Source: CAD feature listing. Evaluate the final solid. Frame: model axes, mm. A direction names the side the tool comes from. Coordinates: 2 decimals unless noted, no trailing zeros. Loops run counter-clockwise (first coordinate to the right, second up) from the corner with the lowest first, then second, coordinate; pieces in that order, holes last. Notation, with made-up numbers: (-12, 21) -> (30, 21) arc R23 cw to (30, 54) -> close; hole circle Ø4 at (21.5, 47). An arc over 180 degrees is marked (long way). Answer as a JSON object with one key per item and string values. Group by question number.
from build123d import *

# Parameters (mm, degrees)
F1_DEPTH = 87.558992
F2_W     = 23.463726
F2_H     = 36.116287
F3_DEPTH = 159.944564


with BuildPart() as f1:
    # F0 (on Top) → F1 (new body)
    with BuildSketch(Plane.XY):
        Polygon((52.528806, 32.23221), (0, 21.399237), (-38.256936, -12.692079), (9.787939, -27.863212), align=None)
    extrude(amount=F1_DEPTH)

    # F2 (on face) → F3 (join)
    with BuildSketch(Plane(origin=(-10.628911, 11.927659, 0), x_dir=(-0.746584, -0.665292, 0), z_dir=(-0.665292, 0.746584, 0))):
        with Locations((9.666294, 53.462007)):
            Rectangle(F2_W, F2_H)
    extrude(amount=F3_DEPTH)


solid = f1.part
1. Mould query, pull axis X, two halves, no side actions, for faces 3 (the face through (26.63, 26.89, 43.17)), 4 (the face through (-70, 64, 35.404)), 5 (the face through (-14.57, -20.17, 43.17)). Classes: pulls with the +X half, pulls with the -X half, needs draft (parallel to the pull), parting line crosses it, or undercut.
2. Section query C-C on y = 62. Return loops of the section in (x, z), then the cut area to 3 significant figures.
3. Pin query (flat end, axial travel): pin 1 Ø5 at (x, z) = (-57.5, 46.5) entering from +Y; pin 2 Ø12 at (y, z) = (12, 35) entering from -X; pin 3 Ø2 at (x, z) = (-27.5, 43.5) entering from +Y. Return the tip coordinate at first contact, or that it passes through.
4. Ray query, L1, parallel to Z at x = -29, y = 10; L2, parallel to Y at x = 11, z = 44; L3, parallel to Y at x = -20, z = 50.5. Return the intervals inside material, ascending.
5. Section query D-D on z = 13.5. Return loops of the section in (x, y).
6. Section query A-A on z = 41.5. Return loops of the section in (x, y).
7. Section query B-B on x = -34. Return loops of the section in (y, z).
8. Reachability of faces 1 (the face through (-70, 64, 71.52)), 2 (the face through (30.859, 1.764, 43.167)) from +Z, -Z, +X, -X, +Y, -Y: full face, straight path, thin tool, end or side. Return the list, or none.
Solved:
{
 "1": {"face 3": "undercut", "face 4": "needs draft", "face 5": "pulls with the -X half"},
 "2": {"outline": "(-83.91, 35.4) -> (-52.48, 35.4) -> (-52.48, 71.52) -> (-83.91, 71.52) -> close", "area": "1,140 mm^2"},
 "3": {"pin 1": "y = 70.44", "pin 2": "x = -44.69", "pin 3": "y = 35.09"},
 "4": {"L1": "35.4 to 71.52", "L2": "-26.16 to 23.67", "L3": "-18.46 to 25.55"},
 "5": {"outline": "(-38.26, -12.69) -> (9.79, -27.86) -> (52.53, 32.23) -> (0, 21.4) -> close"},
 "6": {"outline": "(-133.01, 117.1) -> (-26.6, -2.31) -> (-38.26, -12.69) -> (9.79, -27.86) -> (52.53, 32.23) -> (0, 21.4) -> (-9.09, 13.3) -> (-115.5, 132.71) -> close"},
 "7": {"outline": "(-14.04, 0) -> (-8.9, 0) -> (-8.9, 87.56) -> (-14.04, 87.56) -> close; (5.99, 35.4) -> (41.26, 35.4) -> (41.26, 71.52) -> (5.99, 71.52) -> close"},
 "8": {"face 1": "+Z, -X, +Y", "face 2": "+Z, -Z, +X, -Y"}
}
